Geometry: final body of the model. Coordinates: model frame, mm. A direction names the side the tool comes from. Round coordinates to 2 decimals unless told otherwise and drop trailing zeros. Use a Markdown table: item, result. Add a question column.
```python
from build123d import *

# Parameters (mm, degrees)
SKETCH_R   = 2.1
SKETCH_R_2 = 3.4
PAD_DEPTH  = 500


with BuildPart() as part:
    # Sketch → Pad (new body)
    with BuildSketch(Plane.XY):
        with BuildLine():
            Line((-6, -4.585786), (-6, 4.585786))
            Line((-6, 4.585786), (-9.664214, 8.25))
            Line((-9.664214, 8.25), (-13, 8.25))
            Line((-13, 8.25), (-13, 4))
            Line((-13, 4), (-15, 4))
            Line((-15, 4), (-15, 14))
            ThreePointArc((-14, 15), (-14.707107, 14.707107), (-15, 14))
            Line((-4, 15), (-14, 15))
            Line((-4, 13), (-4, 15))
            Line((-8.25, 13), (-4, 13))
            Line((-8.25, 9.664214), (-8.25, 13))
            Line((-4.585786, 6), (-8.25, 9.664214))
            Line((4.585786, 6), (-4.585786, 6))
            Line((4.585786, 6), (8.25, 9.664214))
            Line((8.25, 9.664214), (8.25, 13))
            Line((8.25, 13), (4, 13))
            Line((4, 13), (4, 15))
            Line((4, 15), (14, 15))
            ThreePointArc((15, 14), (14.707107, 14.707107), (14, 15))
            Line((15, 4), (15, 14))
            Line((13, 4), (15, 4))
            Line((13, 8.25), (13, 4))
            Line((9.664214, 8.25), (13, 8.25))
            Line((6, 4.585786), (9.664214, 8.25))
            Line((6, 4.585786), (6, -4.585786))
            Line((6, -4.585786), (9.664214, -8.25))
            Line((9.664214, -8.25), (13, -8.25))
            Line((13, -8.25), (13, -4))
            Line((13, -4), (15, -4))
            Line((15, -4), (15, -14))
            ThreePointArc((14, -15), (14.707107, -14.707107), (15, -14))
            Line((14, -15), (4, -15))
            Line((4, -15), (4, -13))
            Line((4, -13), (8.25, -13))
            Line((8.25, -13), (8.25, -9.664214))
            Line((8.25, -9.664214), (4.585786, -6))
            Line((4.585786, -6), (-4.585786, -6))
            Line((-4.585786, -6), (-8.25, -9.664214))
            Line((-8.25, -9.664214), (-8.25, -13))
            Line((-8.25, -13), (-4, -13))
            Line((-4, -13), (-4, -15))
            Line((-4, -15), (-14, -15))
            ThreePointArc((-15, -14), (-14.707107, -14.707107), (-14, -15))
            Line((-15, -4), (-15, -14))
            Line((-13, -4), (-15, -4))
            Line((-13, -8.25), (-13, -4))
            Line((-9.664214, -8.25), (-13, -8.25))
            Line((-6, -4.585786), (-9.664214, -8.25))
        make_face()
        with Locations((-11.6, 11.6)):
            Circle(SKETCH_R, mode=Mode.SUBTRACT)
        Circle(SKETCH_R_2, mode=Mode.SUBTRACT)
        with Locations((11.6, 11.6)):
            Circle(SKETCH_R, mode=Mode.SUBTRACT)
        with Locations((-11.6, -11.6)):
            Circle(SKETCH_R, mode=Mode.SUBTRACT)
        with Locations((11.6, -11.6)):
            Circle(SKETCH_R, mode=Mode.SUBTRACT)
    extrude(amount=PAD_DEPTH)


solid = part.part
```
1) Pin query (flat end, axial travel): P1, Ø4, axis at x = -10.5, y = 4, coming from the +Z side; P2, Ø3, axis at x = -1, z = 261, coming from the +Y side. Return the tip coordinate at first contact, or that it passes through.
2) Draft query along Y for faces 4 (the flat face through (-6, 0, 246)), 5 (the flat face through (4, 0, 500)), 6 (the flat face through (-9, -15, 246)). Return one class per face: released by +Y, released by -Y, zero draft, split by the parting line, or undercut.
3) Set-up query: faces 1 (the flat face through (9, -15, 246)), 2 (the flat face through (6, 0, 246)), 3 (the flat face through (9, 15, 246)). Return all of +Z, -Z, +X, -X, +Y, -Y with unobstructed straight access to the full face (end or side cutting, diameter ignored); none if empty.
4) Section A-A, the plane z = 258.5. State how many separate pieces and enclosed holes the cut face has, then the cut area to 3 significant figures.
5) Material intervals for L1, parallel to X at y = -11, z = 134; L2, parallel to Y at x = -11.6, z = 270, sorted ascending. Write a range as from..to.
Output values:
| question | item | result |
|---|---|---|
| 1 | P1 | passes through |
| 1 | P2 | stops at y = 6 |
| 2 | face 4 | undercut |
| 2 | face 5 | zero draft |
| 2 | face 6 | released by -Y |
| 3 | face 1 | +Z, -Z, +X, -X, -Y |
| 3 | face 2 | +Z, -Z |
| 3 | face 3 | +Z, -Z, +X, -X, +Y |
| 4 | separate pieces | 1 |
| 4 | enclosed holes | 5 |
| 4 | area | 335 mm^2 |
| 5 | L1 | x = -15..-13.61, -9.59..-8.25, 8.25..9.59, 13.61..15 |
| 5 | L2 | y = -15..-13.7, -9.5..-8.25, 8.25..9.5, 13.7..15 |
